from build123d import *

# Parameters (mm, degrees)
F0_R     = 10
F1_DEPTH = 41.7
F2_R     = 6.25
F3_DEPTH = 142.3
F5_DEPTH = 9


with BuildPart() as f1:
    # F0 (on Front) → F1 (new body)
    with BuildSketch(Plane.XZ):
        Circle(F0_R)
    extrude(amount=-F1_DEPTH)

    # F2 (on face) → F3 (join)
    with BuildSketch(Plane(origin=(0, 41.7, 0), x_dir=(-1, 0, 0), z_dir=(0, 1, 0))):
        Circle(F2_R)
    extrude(amount=F3_DEPTH)

    # F4 (on face) → F5 (cut)
    with BuildSketch(Plane.XZ):
        Polygon((4.8, -2.771281), (4.8, 2.771281), (0, 5.542563), (-4.8, 2.771281), (-4.8, -2.771281), (0, -5.542563), align=None)
    extrude(amount=-F5_DEPTH, mode=Mode.SUBTRACT)


solid = f1.part
Work out the finished part from the listing and answer in its coordinate system (mm). A direction names the side the tool comes from. Coordinates: 2 decimals unless noted, no trailing zeros. Write each loop counter-clockwise with the first axis right and the second up, starting at its lowest first coordinate (ties: lowest second). Pieces come first, ordered by that corner, then holes.
1. For faces 5 (the flat face through (-2.366, 4.437, 4.176)), 6 (the flat face through (4, 41.7, 5)), 7 (the cylindrical face through (-2.17, 20.56, -9.76)), determine the directions among +Z, -Z, +X, -X, +Y, -Y from which every point of the face is accessible in a straight line to the end or side of a thin tool.
Results list:
face 5: -Y
face 6: +Y
face 7: +Y, -Y
2. For a pull along X with two mould halves and no side action, classify faces 1 (the flat face through (2, 0, 5)), 2 (the flat face through (-4.8, 4, 0)), 3 (the cylindrical face through (-5.96, 111.85, 1.88)), 4 (the flat face through (0, 9, 0)) as +X half, -X half, draft (parallel to the pull), parting line (faces both ways), or undercut.
Results list:
face 1: draft
face 2: undercut
face 3: parting line
face 4: undercut
3. Flat-ended cylindrical pins translate along their axes: pin 1 (3 mm diameter, centred on x = 2, y = 100, fed in from -Z); pin 2 (1.5 mm diameter, centred on y = 121.5, z = -5.5, fed in from -X); pin 3 (4 mm diameter, centred on x = -0.5, z = 1.5, fed in from -Y). Find the tip coordinate at first contact, or state that the pin passes through.
Results list:
pin 1: stops at z = -6.23
pin 2: stops at x = -4.06
pin 3: stops at y = 9
4. The part is cut by section B-B, the plane y = 160.5. Write down the section's boundary in (x, z).
Results list:
outline: circle Ø12.5 at (0, 0)
5. Consider line 1 along Y through (x, z) = (-0.5, 5); line 2 along Y through (x, z) = (7.25, 3); line 3 along X through (y, z) = (125, 0.5). Determine where each line is inside the solid, lowest interval first.
Results list:
line 1: y = 9 to 184
line 2: y = 0 to 41.7
line 3: x = -6.23 to 6.23
6. The part is cut by section A-A, the plane z = 0. Write down the section's boundary in (x, y), and give its area (3 significant figures).
Results list:
outline: (-10, 0) - (-4.8, 0) - (-4.8, 9) - (4.8, 9) - (4.8, 0) - (10, 0) - (10, 41.7) - (6.25, 41.7) - (6.25, 184) - (-6.25, 184) - (-6.25, 41.7) - (-10, 41.7) - close
area: 2,530 mm2
